Autodesk Inventor part; units mm, degrees
ref_plane "YZ Plane" through (0, 0, 0) normal (1, 0, 0) x (0, 1, 0)
ref_plane "XZ Plane" through (0, 0, 0) normal (0, 1, 0) x (-1, 0, 0)
ref_plane "XY Plane" through (0, 0, 0) normal (0, 0, 1) x (1, 0, 0)
sketch "Sketch1" plane through (0, 0, 0) normal (0, 1, 0) x (-1, 0, 0)
  line L0 (-10.4167, 14.023) -> (-62.4167, 14.023)
  line L1 (-62.4167, 14.023) -> (-62.4167, -47.977)
  line L2 (-62.4167, -47.977) -> (-10.4167, -47.977)
  line L3 (-10.4167, -47.977) -> (-10.4167, 14.023)
  circle A0 centre (-64.4167, -45.977) radius 2
  line L4 (-64.4167, -43.977) -> (-62.4167, -43.977)
  line L5 (-64.4167, -47.977) -> (-62.4167, -47.977)
  circle A1 centre (-12.4167, 12.023) radius 2
  circle A2 centre (-12.4167, -45.977) radius 2
  circle A3 centre (-64.4167, 12.023) radius 2
  line L6 (-64.4167, 14.023) -> (-62.4167, 14.023)
  line L7 (-64.4167, 10.023) -> (-62.4167, 10.023)
  point P0 (0, 0)
  point P1 (-10.4167, -45.977)
  point P2 (-10.4167, 12.023)
  point P3 (-12.4167, 14.023)
  point P4 (-12.4167, -47.977)
  dimension "d0" = 52
  dimension "d1" = 62
  dimension "d2" = 4
  dimension "d3" = 2
  dimension "d4" = 2
  dimension "d5" = 4
  dimension "d6" = 4
  dimension "d7" = 4
  dimension "d8" = 2
  dimension "d9" = 2
extrude "Extrusion1" add sketch "Sketch1" along normal blind 1.6 contours A1 L3 A2 L2 L1 L0 | A1 | L1 A3 L6 | A2 | A3 | L1 L7 A3 | L5 A0 L1 | L1 A0 L4 | A0
properties part number "Płytka"
Model file for the job. Use its own axes, mm. A direction names the side the tool comes from. Coordinates: 2 decimals unless noted, no trailing zeros. Write each loop counter-clockwise with the first axis right and the second up, starting at its lowest first coordinate (ties: lowest second). Pieces come first, ordered by that corner, then holes. Notation, with made-up numbers: (-27, -25) - (-17, -25) arc R21 ccw to (-17, -15) - close; hole circle Ø6 at (44, 21.5). An arc over 180 degrees is marked (long way). One line per item, written item: value. Start each with the question number.
1. Flat gauge pin, fed straight in: pin 1 (0.8 mm diameter, centred on y = 0.5, z = -29.5, fed in from +X). Where does the tip first touch, or does it go through?
2. Tool access for faces 1 (the flat face through (63, 1, 10.023)), 2 (the flat face through (10.417, 1, -17)): list every direction of +Z, -Z, +X, -X, +Y, -Y with a clear straight run to the whole face (end or side of a thin tool).
3. Slice it at B-B (z = 3). Write the cut outline in (x, y), plus the area to 3 significant figures.
4. Mould opens along Z. For faces 3 (the cylindrical face through (66.416, 0.789, -46.021)), 4 (the cylindrical face through (66.416, 0.789, 11.979)), 5 (the flat face through (39, 0, -17)), 6 (the flat face through (39, 1, -47.977)) say: released by +Z, released by -Z, zero draft, split by the parting line, or undercut.
5. Slice it at A-A (y = 0.9). Write the cut outline in (x, z).
6. Probe line 1 (X direction, y = 0.3, z = -12). List the from-to ranges inside material, lowest first. Write a range as from..to.
Answers below:
1. pin 1: stops at x = 62.42
2. face 1: +X, +Y, -Y
2. face 2: +Z, -Z, -X, +Y, -Y
3. outline: (10.42, 0) - (62.42, 0) - (62.42, 1.6) - (10.42, 1.6) - close
3. area: 83.2 mm^2
4. face 3: undercut
4. face 4: undercut
4. face 5: zero draft
4. face 6: released by -Z
5. outline: (10.42, -45.98) arc R2 ccw to (12.42, -47.98) - (64.42, -47.98) arc R2 ccw to (64.42, -43.98) - (62.42, -43.98) - (62.42, 10.02) - (64.42, 10.02) arc R2 ccw to (64.42, 14.02) - (12.42, 14.02) arc R2 ccw to (10.42, 12.02) - close
6. line 1: x = 10.42..62.42
